Here's how the part is built. I have some questions about the finished solid (model axes, mm). A direction names the side the tool comes from. Coordinates: 2 decimals unless noted, no trailing zeros. Write each loop counter-clockwise with the first axis right and the second up, starting at its lowest first coordinate (ties: lowest second). Pieces come first, ordered by that corner, then holes. Notation, with made-up numbers: (33.25, 41) - (89.25, 41) arc R11 ccw to (89.25, 55) - close; hole circle Ø4 at (15, 54). An arc over 180 degrees is marked (long way). Answer in a Markdown table with one row per item. Add a question column.
Item 1: I'm going to push flat-ended pins straight in: pin 1 (0.8 mm diameter, centred on x = 8, z = 4, fed in from +Y); pin 2 (2 mm diameter, centred on x = 7.5, z = 3.5, fed in from -Y); pin 3 (1.8 mm diameter, centred on x = 3, z = 1.5, fed in from -Y). Where does each tip first touch, or does it pass through?
Item 2: Which directions (+Z, -Z, +X, -X, +Y, -Y) give clear straight access to the entire face, cutting with the end or side of a thin tool? Please do faces 1 (the face through (3, 4, 3)), 2 (the face through (3.7, 0, 3)), 3 (the face through (-3.02, 10.02, 3.04)).
Item 3: We'd pull the mould along Y, two halves only. Please class faces 4 (the face through (-4.74, 17.27, 2.96)), 5 (the face through (3.8, 12, 3)), 6 (the face through (5.6, 0.2, 0.8)), 7 (the face through (7.115, 10.028, 3.613)): +Y half, -Y half, draft (parallel to the pull), parting line (faces both ways), or undercut.
Item 4: If I drill on probe 1 along Y at (x, z) = (-3.5, 2.75); probe 2 along Y at (x, z) = (-4.5, 5.25); probe 3 along Y at (x, z) = (4, 5.75), over which ranges is the centre line in solid material (lowest first)? Write a range as from..to.
Item 5: Imagine slicing it at D-D (z = 1). Please give me the cut outline in (x, y), plus the area to 3 significant figures.
Item 6: Imagine slicing it at C-C (x = 2). Please give me the cut outline in (y, z).
Item 7: Imagine slicing it at B-B (y = -5). Please give me the cut outline in (x, z), plus the area to 3 significant figures.
Item 8: Imagine slicing it at A-A (z = 3.5). Please give me the cut outline in (x, y), plus the area to 3 significant figures.
Autodesk Inventor part; units mm, degrees
ref_plane "YZ Plane" through (0, 0, 0) normal (1, 0, 0) x (0, 1, 0)
ref_plane "XZ Plane" through (0, 0, 0) normal (0, 1, 0) x (-1, 0, 0)
ref_plane "XY Plane" through (0, 0, 0) normal (0, 0, 1) x (1, 0, 0)
sketch "スケッチ1" plane through (0, 0, 0) normal (0, 0, 1) x (1, 0, 0)
  line L0 (9, 0) -> (9, 4)
  line L1 (9, 12) -> (2.2731, 12)
  line L2 (0, 8) -> (9, 8)
  line L3 (0, 4) -> (9, 4)
  line L4 (9, 8) -> (9, 12)
  arc A0 (0, 8) -> (0, 4) centre (-5.7099, 6) ccw
  line L5 (2.2731, 12) -> (0, 14.2779)
  line L6 (2.2731, 0) -> (-5.7099, -8)
  line L7 (-5.7099, 20) -> (-15.7099, 20)
  line L8 (-5.7099, -8) -> (-15.7099, -8)
  line L9 (-15.7099, 20) -> (-25.7698, 20)
  line L10 (-25.7698, 20) -> (-25.7698, -8)
  line L11 (-25.7698, -8) -> (-15.7099, -8)
  line L12 (2.2731, 0) -> (9, 0)
  line L13 (0, 14.2779) -> (-5.7099, 20)
  point P0 (0, 0)
  point P1 (4.5, 12)
  point P2 (4.5, 0)
  point P3 (4.5, 4)
  point P4 (-25.7099, 6)
  dimension "d4" = 12.1
  dimension "d5" = 4
  dimension "d6" = 14
  dimension "d7" = 14
  dimension "d8" = 10
  dimension "d9" = 10
  dimension "d10" = 20
  dimension "d12" = 14
extrude "押し出し1" add sketch "スケッチ1" along normal blind 6
sketch "スケッチ2" plane through (0, 0, 6) normal (0, 0, 1) x (1, 0, 0)
  circle A0 centre (5.6365, 13.3) radius 1.5
  line L0 (9, 8) -> (9, 12)
  line L1 (11.5477, 6) -> (-28.1936, 6) construction
  line L2 (9, 12) -> (2.2731, 12)
  circle A1 centre (5.6365, -1.3) radius 1.5
  point P0 (0, 0)
  point P1 (4.8882, 12)
  point P2 (6.3849, 12)
  dimension "d15" = 3
  dimension "d16" = 3.3635
  dimension "d17" = 1.3
extrude "押し出し2" cut sketch "スケッチ2" against normal blind 6 contours A0 L2 | A1 picked at (5.4614, 13.0013)
sketch "スケッチ3" plane through (0, 0, 6) normal (0, 0, 1) x (1, 0, 0)
  circle A0 centre (5.6365, 13.3) radius 1.5
  line L0 (9, 12) -> (2.2731, 12)
  point P0 (0, 0)
  point P1 (4.8882, 12)
  point P2 (6.3849, 12)
  dimension "d20" = 3
  dimension "d21" = 1.3
extrude "押し出し3" add sketch "スケッチ3" against normal blind 6 contours A0 L0 picked at (5.4614, 13.0013)
sketch "スケッチ4" plane through (0, 0, 6) normal (0, 0, 1) x (1, 0, 0)
  arc A0 (6.3849, 12) -> (4.8882, 12) centre (5.6365, 13.3) ccw
  circle A1 centre (5.6365, 13.3) radius 1.5
  point P0 (0, 0)
  dimension "d24" = 3
extrude "押し出し4" cut sketch "スケッチ4" against normal blind 6
fillet "フィレット1" radius 5 1 edges at (-25.7698, 20, 3)
fillet "フィレット2" radius 5 1 edges at (-25.7698, -8, 3)
fillet "フィレット3" radius 3 4 edges at (-5.7099, -8, 3) (2.2731, 0, 3) (-5.7099, 20, 3) (2.2731, 12, 3)
sketch "スケッチ6" plane through (0, 4, 0) normal (0, 1, 0) x (1, 0, 0)
  point P0 (0, 0)
sketch "スケッチ7" plane through (4.8882, 12, 6) normal (0, 1, 0) x (1, 0, 0)
  circle A0 centre (0.7488, 3) radius 1.6
  line L0 (1.4967, 0) -> (0, 0)
  line L1 (4.1118, 6) -> (4.1118, 0)
  point P0 (-4.8882, 6)
  point P1 (0.7483, 0)
  dimension "d43" = 3.2
  dimension "d44" = 3
  dimension "d45" = 3.363
extrude "押し出し5" cut sketch "スケッチ7" against normal blind 28
sketch "スケッチ11" plane through (0, 0, 6) normal (0, 0, 1) x (1, 0, 0)
  line L0 (-6.9544, 20) -> (-20.7698, 20)
  line L1 (-20.7698, 20) -> (-6.9544, 20)
  arc A0 (1.394, 12.8809) -> (3.5176, 12) centre (3.5176, 15) ccw
  line L2 (0, 20) -> (1.3068, 17.0279)
  arc A1 (1.394, 12.8809) -> (3.5176, 12) centre (3.5176, 15) ccw
  arc A2 (-4.8308, 19.1191) -> (-6.9544, 20) centre (-6.9544, 17) ccw
  arc A3 (-4.8308, 19.1191) -> (-6.9544, 20) centre (-6.9544, 17) ccw
  line L3 (1.394, 12.8809) -> (-4.8308, 19.1191)
  line L4 (-4.8308, 19.1191) -> (1.394, 12.8809)
  arc A4 (0, 8) -> (0, 4) centre (-5.7099, 6) ccw
  line L5 (-11.7599, 6) -> (12.1155, 6) construction
  line L6 (-20.7698, -8) -> (0, -8)
  line L7 (0, -8) -> (3.5176, 0)
  arc A5 (-6.9544, -8) -> (-4.8308, -7.1191) centre (-6.9544, -5) ccw
  line L8 (1.394, -0.8809) -> (-4.8308, -7.1191)
  line L9 (-6.9544, 20) -> (0, 20)
  line L10 (1.3068, 17.0279) -> (3.5176, 12)
  arc A6 (3.5176, 0) -> (1.394, -0.8809) centre (3.5176, -3) ccw
  point P0 (0, 0)
extrude "押し出し6" add sketch "スケッチ11" against normal blind 6
sketch "スケッチ12" plane through (0, 0, 6) normal (0, 0, 1) x (1, 0, 0)
  arc A0 (0, 8) -> (0, 4) centre (-5.7099, 6) ccw
  point P0 (0, 0)
  point P1 (-15.7099, 6)
  point P2 (-5.7099, 16)
  point P3 (-5.7099, -4)
  dimension "d74" = 10
  dimension "d76" = 10
  dimension "d77" = 10
hole "穴4" at (-15.7099, 6, 6) at (-5.7099, 16, 6) at (-5.7099, -4, 6) direction (0, 0, -1) diameter 3.2 end through all
sketch "スケッチ13" plane through (0, 0, 6) normal (0, 0, 1) x (1, 0, 0)
  line L0 (-20.7698, -8) -> (0, -8)
  line L1 (0, 20) -> (-20.7698, 20)
  line L2 (-18.7698, 20) -> (-18.7698, -8) construction
  line L3 (-25.7698, 15) -> (-25.7698, -3)
  arc A0 (-18.7698, 20) -> (-18.7698, -8) centre (6.3784, 6) ccw
  line L4 (-18.7698, 20) -> (-29.3351, 20)
  line L5 (-29.3351, 20) -> (-29.3351, -8)
  line L6 (-29.3351, -8) -> (-18.7698, -8)
  point P0 (0, 0)
  dimension "d85" = 7
extrude "押し出し7" cut sketch "スケッチ13" against normal blind 6
fillet "フィレット4" radius 6 1 edges at (-18.7698, 20, 3)
fillet "フィレット5" radius 6 1 edges at (-18.7698, -8, 3)
sketch "スケッチ14" plane through (0, 0, 6) normal (0, 0, 1) x (1, 0, 0)
  arc A0 (0, 8) -> (0, 4) centre (-3.5217, 6) ccw
  arc A1 (0, 8) -> (0, 4) centre (-5.7099, 6) ccw
  point P0 (0, 0)
  point P1 (0, 4)
  dimension "d90" = 8.1
extrude "押し出し8" add sketch "スケッチ14" against normal blind 6
sketch "スケッチ15" plane through (0, 0, 6) normal (0, 0, 1) x (1, 0, 0)
  arc A0 (0, 8) -> (0, 4) centre (-3.5217, 6) ccw
  line L0 (-6.5217, 3.2792) -> (-6.5217, 8.7208)
  point P0 (0, 0)
  point P1 (-6.5217, 6)
  dimension "d93" = 3
extrude "押し出し9" add sketch "スケッチ15" against normal blind 6
properties part number "射出_腕固定3" material "ポリカーボネート、クリア"
Here are the results:
| question | item | result |
|---|---|---|
| 1 | pin 1 | stops at y = 12 |
| 1 | pin 2 | stops at y = 0 |
| 1 | pin 3 | stops at y = -3.22 |
| 2 | face 1 | +Z, -Z, +X |
| 2 | face 2 | +Z, -Z, +X, -Y |
| 2 | face 3 | +Z, -Z |
| 3 | face 4 | undercut |
| 3 | face 5 | +Y half |
| 3 | face 6 | -Y half |
| 3 | face 7 | draft |
| 4 | probe 1 | y = -8..1.95, 10.05..20 |
| 4 | probe 2 | y = -8..-5.05, -2.95..2.07, 9.93..14.95, 17.05..20 |
| 4 | probe 3 | y = 0..4, 8..12 |
| 5 | outline | (-20.57, -4.11) arc R6 ccw to (-14.95, -8) - (0, -8) - (3.52, 0) - (4.89, 0) arc R1.5 cw to (6.38, 0) - (9, 0) - (9, 4) - (0, 4) arc R4.05 cw to (-6.52, 3.28) - (-6.52, 8.72) arc R4.05 cw to (0, 8) - (9, 8) - (9, 12) - (6.38, 12) arc R1.5 cw to (4.89, 12) - (3.52, 12) - (1.31, 17.03) - (0, 20) - (-14.95, 20) arc R6 ccw to (-20.57, 16.11) arc R28.78 ccw to start; hole circle Ø3.2 at (-15.71, 6); hole circle Ø3.2 at (-5.71, -4); hole circle Ø3.2 at (-5.71, 16) |
| 5 | area | 618 mm2 |
| 6 | outline | (-3.45, 0) - (4, 0) - (4, 6) - (-3.45, 6) - close; (8, 0) - (15.45, 0) - (15.45, 6) - (8, 6) - close |
| 7 | outline | (-20.15, 0) - (-6.96, 0) - (-6.96, 6) - (-20.15, 6) - close; (-4.46, 0) - (1.32, 0) - (1.32, 6) - (-4.46, 6) - close |
| 7 | area | 114 mm2 |
| 8 | outline | (-20.57, -4.11) arc R6 ccw to (-14.95, -8) - (0, -8) - (3.52, 0) - (4.12, 0) - (4.12, 4) - (0, 4) arc R4.05 cw to (-6.52, 3.28) - (-6.52, 8.72) arc R4.05 cw to (0, 8) - (4.12, 8) - (4.12, 12) - (3.52, 12) - (1.31, 17.03) - (0, 20) - (-14.95, 20) arc R6 ccw to (-20.57, 16.11) arc R28.78 ccw to start; (7.16, 0) - (9, 0) - (9, 4) - (7.16, 4) - close; (7.16, 8) - (9, 8) - (9, 12) - (7.16, 12) - close; hole circle Ø3.2 at (-15.71, 6); hole circle Ø3.2 at (-5.71, -4); hole circle Ø3.2 at (-5.71, 16) |
| 8 | area | 594 mm2 |
